Read the model definition and answer for the solid it produces. Units are mm, in the model's axes. Give positions to 0.01 mm unless a question says otherwise; leave off trailing zeros. Loops run counter-clockwise (first coordinate to the right, second up) from the corner with the lowest first, then second, coordinate; pieces in that order, holes last. Notation, with made-up numbers: (85, 84.25) - (99, 84.25) arc R35 cw to (99, 117.25) - close; hole circle Ø10 at (4.5, -33.5). An arc over 180 degrees is marked (long way). Write item = value, one per line.
```python
from build123d import *

# Parameters (mm, degrees)
F0_R           = 1.27
F1_DEPTH       = 12.7
F3_D           = 15.875
F5_D           = 16.66748
F5_CSINK_D     = 30.1752
F5_CSINK_ANGLE = 82
F7_D           = 12.7


# Not quite as in the source:
# - a feature names something its author has since deleted; it is built from what else it names


with BuildPart() as f1:
    # F0 (on Top) → F1 (new body)
    with BuildSketch(Plane.XY):
        Polygon((-2.5901260614, -38.4407882191), (-2.5901260614, 12.3592117809), (-2.5901260614, 63.1592117809), (-2.5901260614, 75.8592117809), (-104.1901260614, 75.8592117809), (-104.1901260614, 63.1592117809), (-104.1901260614, -38.4407882191), align=None)
        with Locations((-85.1401260614, 12.3592117809)):
            Circle(F0_R, mode=Mode.SUBTRACT)
        with Locations((-78.4163327398, -7.1792497576)):
            Circle(F0_R, mode=Mode.SUBTRACT)
        with Locations((-53.3901260614, -19.3907882191)):
            Circle(F0_R, mode=Mode.SUBTRACT)
        with Locations((-53.3901260614, 12.3592117809)):
            Circle(F0_R, mode=Mode.SUBTRACT)
        with Locations((-23.1804483045, 2.5899810116)):
            Circle(F0_R, mode=Mode.SUBTRACT)
        with BuildLine():
            ThreePointArc((-13.3851260614, 12.3592117809), (-12.1151260614, 13.6292117809), (-10.8451260614, 12.3592117809))
            ThreePointArc((-10.8451260614, 12.3592117809), (-12.1151260614, 11.0892117809), (-13.3851260614, 12.3592117809))
        make_face(mode=Mode.SUBTRACT)
        with Locations((-92.6627071454, 25.0592117809)):
            Circle(F0_R, mode=Mode.SUBTRACT)
        with Locations((-20.8560573795, 37.7592117809)):
            Circle(F0_R, mode=Mode.SUBTRACT)
        with Locations((-53.3901260614, 53.6342117809)):
            Circle(F0_R, mode=Mode.SUBTRACT)
        with Locations((-92.6627071454, 25.0592117809)):
            Circle(F0_R)
        with Locations((-85.1401260614, 12.3592117809)):
            Circle(F0_R)
        with Locations((-78.4163327398, -7.1792497576)):
            Circle(F0_R)
        with Locations((-23.1804483045, 2.5899810116)):
            Circle(F0_R)
        with Locations((-20.8560573795, 37.7592117809)):
            Circle(F0_R)
        with BuildLine():
            ThreePointArc((-13.3851260614, 12.3592117809), (-12.1151260614, 11.0892117809), (-10.8451260614, 12.3592117809))
            Line((-10.8451260614, 12.3592117809), (-13.3851260614, 12.3592117809))
        make_face()
        with BuildLine():
            Line((-13.3851260614, 12.3592117809), (-10.8451260614, 12.3592117809))
            ThreePointArc((-10.8451260614, 12.3592117809), (-12.1151260614, 13.6292117809), (-13.3851260614, 12.3592117809))
        make_face()
    extrude(amount=F1_DEPTH)

    # F3 (through all)
    with Locations(Plane.XY.offset(12.7)):
        with Locations((-53.3901260614, 12.3592117809)):
            Hole(F3_D / 2)

    # F5 (through all)
    with Locations(Plane(origin=(0, 0, 0), x_dir=(1, 0, 0), z_dir=(0, 0, -1))):
        with Locations((-53.3901260614, -53.6342117809)):
            CounterSinkHole(F5_D / 2, F5_CSINK_D / 2, counter_sink_angle=F5_CSINK_ANGLE)

    # F7 (through all)
    with Locations(Plane.XY.offset(12.7)):
        with Locations((-53.3901260614, -19.3907882191)):
            Hole(F7_D / 2)


solid = f1.part
```
1) This flat-tipped pin is pushed along its axis until it touches: P1, Ø12, axis at x = -43, y = -13, coming from the -Z side. Where does it stop, or does it pass through?
Output:
P1 = 0
2) A cutting plane is placed at A-A on y = 8. Determine the outline of the cut face in (x, z).
Output:
outline = (-104.19, 0) - (-60.02, 0) - (-60.02, 12.7) - (-104.19, 12.7) - close; (-46.76, 0) - (-2.59, 0) - (-2.59, 12.7) - (-46.76, 12.7) - close
3) The mould has two halves that part along X. Classify faces 1 (the face through (-62, 51, 7)), 2 (the face through (-65, 20, 12.7)), 3 (the face through (-2.59, 18, 6)): pulls with the +X half, pulls with the -X half, needs draft (parallel to the pull), parting line crosses it, or undercut.
Output:
face_1 = undercut
face_2 = needs draft
face_3 = pulls with the +X half
4) Find the intervals of material crossed by probe 1 along X at (y, z) = (11, 11.5); probe 2 along X at (y, z) = (53, 2.5); probe 3 along Y at (x, z) = (-63, 3.75), in increasing order.
Output:
probe_1 = -104.19 to -61.21, -45.57 to -2.59
probe_2 = -104.19 to -66.29, -40.49 to -2.59
probe_3 = -38.44 to 46.74, 60.53 to 75.86
5) A cutting plane is placed at B-B on z = 2. Give the number of separate pieces and of enclosed holes in the cut face, then the cut area to 3 significant figures.
Output:
separate_pieces = 1
enclosed_holes = 3
area = 10,700 mm²
